The listing builds one solid part. Answer for the finished solid, in the listing's coordinates (mm). Coordinates: 2 decimals unless noted, no trailing zeros. Order: outer loops, then holes, each group sorted by start corner. A loop starts at its lowest first (then second) coordinate and runs counter-clockwise, first axis right, second up. Notation, with made-up numbers: (8, -31.5) -> (47, -31.5) arc R30 ccw to (47, 4.5) -> close; hole circle Ø1 at (86.5, 72.5). An arc over 180 degrees is marked (long way). Answer in a Markdown table with one row per item. Add a question column.
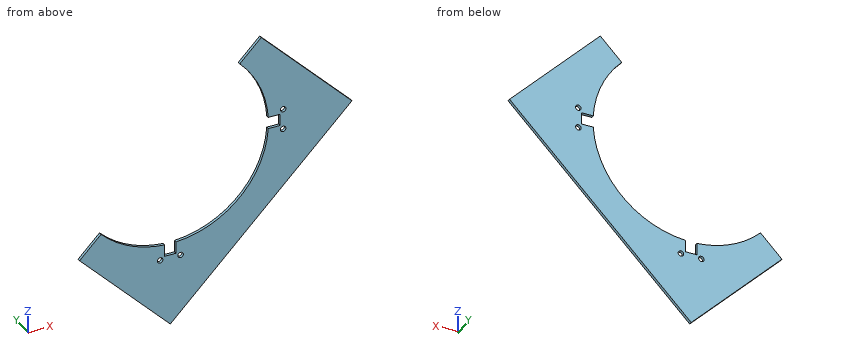
```python
from build123d import *

# Parameters (mm, degrees)
SKETCH1_R           = 1.5
SKETCH1_R_2         = 53.34
BOSS_EXTRUDE1_DEPTH = 1.5875
CUT_EXTRUDE3_DEPTH  = 140.70900378
CUT_EXTRUDE4_DEPTH  = 140.70900378


with BuildPart() as part:
    # Sketch1 → Boss-Extrude1 (new body)
    with BuildSketch(Plane(origin=(0, 0, 0), x_dir=(1, 0, 0), z_dir=(0, 1, 0))):
        Polygon((0.047005036, -98.782806148), (-98.782806148, -0.047005036), (-0.047005036, 98.782806148), (98.782806148, 0.047005036), align=None)
        with Locations(Location((-61.346730494, 5.55625, 0), (0, 0, 270))):
            Circle(SKETCH1_R, mode=Mode.SUBTRACT)
        with Locations(Location((-61.346730494, -5.55625, 0), (0, 0, 270))):
            Circle(SKETCH1_R, mode=Mode.SUBTRACT)
        with Locations(Location((-5.55625, -61.346730494, 0), (0, 0, 270))):
            Circle(SKETCH1_R, mode=Mode.SUBTRACT)
        with Locations(Location((5.55625, -61.346730494, 0), (0, 0, 270))):
            Circle(SKETCH1_R, mode=Mode.SUBTRACT)
        with Locations(Location((61.346730494, -5.55625, 0), (0, 0, 270))):
            Circle(SKETCH1_R, mode=Mode.SUBTRACT)
        with Locations(Location((61.346730494, 5.55625, 0), (0, 0, 270))):
            Circle(SKETCH1_R, mode=Mode.SUBTRACT)
        with Locations(Location((5.55625, 61.346730494, 0), (0, 0, 270))):
            Circle(SKETCH1_R, mode=Mode.SUBTRACT)
        with Locations(Location((-5.55625, 61.346730494, 0), (0, 0, 270))):
            Circle(SKETCH1_R, mode=Mode.SUBTRACT)
        with Locations(Location((0, 0, 0), (0, 0, 270))):
            Circle(SKETCH1_R_2, mode=Mode.SUBTRACT)
    extrude(amount=BOSS_EXTRUDE1_DEPTH)

    # Sketch2 → Cut-Extrude3 (cut, through all)
    with BuildSketch(Plane(origin=(0, 1.5875, 0), x_dir=(1, 0, 0), z_dir=(0, 1, 0))):
        Polygon((3.175, 53.34), (3.175, 59.69), (-3.175, 59.69), (-3.175, 53.34), (-3.175, 52.244537665), (3.175, 52.244537665), align=None)
        Polygon((53.34, -3.175), (59.69, -3.175), (59.69, 3.175), (53.34, 3.175), (52.244537665, 3.175), (52.244537665, -3.175), align=None)
        Polygon((-3.175, -53.34), (-3.175, -59.69), (3.175, -59.69), (3.175, -53.34), (3.175, -52.244537665), (-3.175, -52.244537665), align=None)
        Polygon((-53.34, 3.175), (-59.69, 3.175), (-59.69, -3.175), (-53.34, -3.175), (-52.244537665, -3.175), (-52.244537665, 3.175), align=None)
    extrude(amount=-CUT_EXTRUDE3_DEPTH, mode=Mode.SUBTRACT)

    # Sketch3 → Cut-Extrude4 (cut, through all)
    with BuildSketch(Plane(origin=(0, 1.5875, 0), x_dir=(1, 0, 0), z_dir=(0, 1, 0))):
        Polygon((-49.414905592, 49.367900556), (49.414905592, -49.367900556), (0.047005036, -98.782806148), (-98.782806148, -0.047005036), align=None)
    extrude(amount=-CUT_EXTRUDE4_DEPTH, mode=Mode.SUBTRACT)


solid = part.part
```
Q1. A cutting plane is placed at B-B (y = 0.5). Determine the outline of the cut face in (x, z) (3 decimals), then the cut area to 3 significant figures.
Q2. Straight lines are drawn through the part: line 1 (Z direction, x = 46.5, y = 0.6); line 2 (X direction, y = 0.85, z = -58.5) (1 decimal); line 3 (X direction, y = 0.85, z = 11). For each, find the intervals that lie inside material, in ascending order.
Q3. Given pin 1 (1.8 mm diameter, centred on x = 5.56, z = -61.35, fed in from -Y); pin 2 (0.5 mm diameter, centred on y = 1, z = -56, fed in from +X); pin 3 (0.5 mm diameter, centred on y = 0.5, z = -55.5, fed in from -X); pin 4 (0.5 mm diameter, centred on x = 56, y = 0.5, fed in from +Z), each flat-ended and moving along its own axis, determine where each tip first touches the part or whether it passes through.
Q4. A cutting plane is placed at C-C (x = -26). Determine the outline of the cut face in (y, z), then the cut area to 3 significant figures.
Q5. A cutting plane is placed at D-D (z = -18.5). Determine the outline of the cut face in (x, y).
Q6. A cutting plane is placed at A-A (z = -46). Determine the outline of the cut face in (x, y).
Returned:
| question | item | result |
|---|---|---|
| 1 | outline | (-49.415, -49.368) -> (-0.047, -98.783) -> (98.783, -0.047) -> (49.415, 49.368) -> (37.735, 37.699) arc R53.34 cw to (53.245, 3.175) -> (59.69, 3.175) -> (59.69, -3.175) -> (53.245, -3.175) arc R53.34 cw to (3.175, -53.245) -> (3.175, -59.69) -> (-3.175, -59.69) -> (-3.175, -53.245) arc R53.34 cw to (-37.735, -37.699) -> close; hole circle Ø3 at (-5.556, -61.347); hole circle Ø3 at (5.556, -61.347); hole circle Ø3 at (61.347, -5.556); hole circle Ø3 at (61.347, 5.556) |
| 1 | area | 5,180 mm² |
| 2 | line 1 | z = -52.28 to -26.13, 26.13 to 46.46 |
| 2 | line 2 | x = -40.3 to -3.2, 3.2 to 40.3 |
| 2 | line 3 | x = 52.19 to 87.75 |
| 3 | pin 1 | passes through |
| 3 | pin 2 | stops at x = 43.03 |
| 3 | pin 3 | stops at x = -43.54 |
| 3 | pin 4 | stops at z = 43.03 |
| 4 | outline | (0, -72.81) -> (1.59, -72.81) -> (1.59, -46.57) -> (0, -46.57) -> close |
| 4 | area | 41.6 mm² |
| 5 | outline | (50.03, 0) -> (80.31, 0) -> (80.31, 1.59) -> (50.03, 1.59) -> close |
| 6 | outline | (-46.04, 0) -> (-27, 0) -> (-27, 1.59) -> (-46.04, 1.59) -> close; (27, 0) -> (52.79, 0) -> (52.79, 1.59) -> (27, 1.59) -> close |
